Geometry check sheet. Reference: the model listing, model coordinates, mm. A direction names the side the tool comes from. Give positions to 0.01 mm unless a question says otherwise; leave off trailing zeros. Loops run counter-clockwise (first coordinate to the right, second up) from the corner with the lowest first, then second, coordinate; pieces in that order, holes last. Notation, with made-up numbers: (29.5, -23.75) - (48.5, -23.75) arc R25 cw to (48.5, 14.25) - close; hole circle Ø10 at (4, -36). An arc over 180 degrees is marked (long way). One line per question, with ' | ' between items. Start each with the question number.
from build123d import *

# Parameters (mm, degrees)
SKETCH2_W           = 46.7
SKETCH2_H           = 91
SKETCH2_R           = 1
SKETCH2_W_2         = 26.073503968
SKETCH2_H_2         = 16.277986644
BOSS_EXTRUDE1_DEPTH = 3


with BuildPart() as part:
    # Sketch2 → Boss-Extrude1 (new body)
    with BuildSketch(Plane.XY):
        Rectangle(SKETCH2_W, SKETCH2_H)
        with Locations((17.675, 35)):
            Circle(SKETCH2_R, mode=Mode.SUBTRACT)
        with Locations(Location((-17.675, 35, 0), (0, 0, 180))):
            Circle(SKETCH2_R, mode=Mode.SUBTRACT)
        with Locations((-17.675, -35)):
            Circle(SKETCH2_R, mode=Mode.SUBTRACT)
        with Locations(Location((17.675, -35, 0), (0, 0, 180))):
            Circle(SKETCH2_R, mode=Mode.SUBTRACT)
        with Locations((0, -18.185085705)):
            Rectangle(SKETCH2_W_2, SKETCH2_H_2, mode=Mode.SUBTRACT)
    extrude(amount=BOSS_EXTRUDE1_DEPTH)


solid = part.part
(1) Section check A-A, the plane y = 35. Record the boundary of the cut face in (x, z) (3 decimals), and give its area (3 significant figures).
(2) Section check B-B, the plane y = -18.5. Record the boundary of the cut face in (x, z).
(3) Section check C-C, the plane x = 4.5. Record the boundary of the cut face in (y, z).
(4) Section check D-D, the plane z = 2.05. Record the boundary of the cut face in (x, y) (3 decimals).
(5) Material ranges on line 1 (Y direction, x = 0.5, z = 1.6); line 2 (Y direction, x = -17.5, z = 0.45); line 3 (Y direction, x = -18, z = 0.7), recorded low to high.
(6) Tool access check on faces 1 (the face through (0, 1, 0)), 2 (the face through (-13.037, -18, 1)). Record the directions out of +Z, -Z, +X, -X, +Y, -Y that give a thin tool (end or side, any length) a straight path to the whole face; none if there is none.
Numbers:
1) outline: (-23.35, 0) - (-18.675, 0) - (-18.675, 3) - (-23.35, 3) - close; (-16.675, 0) - (16.675, 0) - (16.675, 3) - (-16.675, 3) - close; (18.675, 0) - (23.35, 0) - (23.35, 3) - (18.675, 3) - close | area: 128 mm^2
2) outline: (-23.35, 0) - (-13.04, 0) - (-13.04, 3) - (-23.35, 3) - close; (13.04, 0) - (23.35, 0) - (23.35, 3) - (13.04, 3) - close
3) outline: (-45.5, 0) - (-26.32, 0) - (-26.32, 3) - (-45.5, 3) - close; (-10.05, 0) - (45.5, 0) - (45.5, 3) - (-10.05, 3) - close
4) outline: (-23.35, -45.5) - (23.35, -45.5) - (23.35, 45.5) - (-23.35, 45.5) - close; hole circle Ø2 at (-17.675, -35); hole circle Ø2 at (-17.675, 35); hole (-13.037, -26.324) - (13.037, -26.324) - (13.037, -10.046) - (-13.037, -10.046) - close; hole circle Ø2 at (17.675, -35); hole circle Ø2 at (17.675, 35)
5) line 1: -45.5 to -26.32, -10.05 to 45.5 | line 2: -45.5 to -35.98, -34.02 to 34.02, 35.98 to 45.5 | line 3: -45.5 to -35.95, -34.05 to 34.05, 35.95 to 45.5
6) face 1: -Z, +X, -X, +Y, -Y | face 2: +Z, -Z
